Check sheet for the modelled part. Datum: model origin and axes. Units: mm. A direction names the side the tool comes from. Round coordinates to 2 decimals unless told otherwise and drop trailing zeros. Write each loop counter-clockwise with the first axis right and the second up, starting at its lowest first coordinate (ties: lowest second). Pieces come first, ordered by that corner, then holes. Notation, with made-up numbers: (52, 11) -> (82, 11) arc R21 ccw to (82, 44) -> close; hole circle Ø11 at (-37, 85.5). An arc over 180 degrees is marked (long way). Write item = value, one per line.
Autodesk Inventor part; units mm, degrees
ref_plane "YZ Plane" through (0, 0, 0) normal (1, 0, 0) x (0, 1, 0)
ref_plane "XZ Plane" through (0, 0, 0) normal (0, 1, 0) x (-1, 0, 0)
ref_plane "XY Plane" through (0, 0, 0) normal (0, 0, 1) x (1, 0, 0)
sketch "Sketch1" plane through (0, 0, 0) normal (0, 1, 0) x (-1, 0, 0)
  line L0 (-9.45, 13.9) -> (9.45, 13.9)
  line L1 (9.45, 13.9) -> (9.45, 12.4)
  line L2 (9.45, 12.4) -> (-9.45, 12.4)
  line L3 (-9.45, 12.4) -> (-9.45, 13.9)
  line L4 (9.45, 12.4) -> (6.45, 12.4)
  line L5 (6.45, 12.4) -> (6.45, -9)
  line L6 (6.45, -9) -> (9.45, -9)
  line L7 (9.45, -9) -> (9.45, 12.4)
  line L8 (-9.45, 12.4) -> (-7.95, 12.4)
  line L9 (-7.95, 12.4) -> (-7.95, -9)
  line L10 (-7.95, -9) -> (-9.45, -9)
  line L11 (-9.45, -9) -> (-9.45, 12.4)
  line L12 (-7.95, -7.6) -> (-9.45, -7.6)
  line L13 (-9.45, -7.6) -> (-9.45, -10.6)
  line L14 (-9.45, -10.6) -> (-7.95, -10.6)
  line L15 (-7.95, -10.6) -> (-7.95, -7.6)
  line L16 (1.45, -9) -> (9.45, -9)
  line L17 (9.45, -9) -> (9.45, -12)
  line L18 (9.45, -12) -> (1.45, -12)
  line L19 (1.45, -12) -> (1.45, -9)
  line L20 (-9.45, -10.6) -> (-7.95, -10.6)
  line L21 (-7.95, -10.6) -> (-7.95, -27.6)
  line L22 (-7.95, -27.6) -> (-9.45, -27.6)
  line L23 (-9.45, -27.6) -> (-9.45, -10.6)
  line L24 (9.45, -12) -> (6.45, -12)
  line L25 (6.45, -12) -> (6.45, -27.6)
  line L26 (6.45, -27.6) -> (9.45, -27.6)
  line L27 (9.45, -27.6) -> (9.45, -12)
  line L28 (-7.95, -27.6) -> (-19.45, -27.6)
  line L29 (-19.45, -27.6) -> (-19.45, -30.6)
  line L30 (-19.45, -30.6) -> (-7.95, -30.6)
  line L31 (-7.95, -30.6) -> (-7.95, -27.6)
  line L32 (6.45, -27.6) -> (19.45, -27.6)
  line L33 (19.45, -27.6) -> (19.45, -30.6)
  line L34 (19.45, -30.6) -> (6.45, -30.6)
  line L35 (6.45, -30.6) -> (6.45, -27.6)
  line L36 (-14.45, -26) -> (-14.45, -42) construction
  line L37 (14.45, -27) -> (14.45, -42) construction
  point P0 (0, 0)
  point P1 (0, 12.4)
  dimension "d0" = 1.5
  dimension "d1" = 3
  dimension "d2" = 1.5
  dimension "d3" = 3
  dimension "d4" = 3
  dimension "d5" = 0
  dimension "d6" = 5
  dimension "d7" = 14.4
  dimension "d8" = 21.4
  dimension "d9" = 20
  dimension "d12" = 0
  dimension "d13" = 0
  dimension "d20" = 17
  dimension "d21" = 10
  dimension "d22" = 1.5
  dimension "d23" = 3
  dimension "d24" = 10
  dimension "d25" = 3
  dimension "d26" = 3
  dimension "d33" = 5
  dimension "d34" = 5
  dimension "d35" = 28.9
extrude "Extrusion1" add sketch "Sketch1" along normal blind 10
sketch "Sketch6" plane through (19.45, 0, -30.6) normal (0, 0, -1) x (-1, 0, 0)
  line L0 (0, 10) -> (11.5, 10)
  line L1 (0, 0) -> (10, 0)
  line L2 (10, 0) -> (10, 10)
  line L3 (10, 10) -> (0, 10)
  line L4 (0, 10) -> (0, 0)
  circle A0 centre (5, 5) radius 2.25
  point P0 (19.45, 0)
  dimension "d27" = 4.5
sketch "Sketch7" plane through (-6.45, 0, -30.6) normal (0, 0, -1) x (-1, 0, 0)
  line L0 (0, 10) -> (13, 10)
  line L1 (13, 0) -> (3, 0)
  line L2 (3, 0) -> (3, 10)
  line L3 (3, 10) -> (13, 10)
  line L4 (13, 10) -> (13, 0)
  circle A0 centre (8, 5) radius 2.25
  point P0 (-6.45, 0)
  dimension "d28" = 4.5
extrude "Extrusion4" cut sketch "Sketch6" against normal blind 4 contours A0
extrude "Extrusion5" cut sketch "Sketch7" against normal blind 4 contours A0
sketch "Sketch8" plane through (0, 0, 0) normal (0, -1, 0) x (1, 0, 0)
  line L0 (2.9056, 16.2719) -> (14.45, 16.2719)
  line L1 (14.45, 16.2719) -> (14.45, -17.7657)
  line L2 (14.45, -17.7657) -> (2.9056, -17.7657)
  line L3 (2.9056, -17.7657) -> (2.9056, 16.2719)
  point P0 (0, 0)
extrude "Extrusion6" cut sketch "Sketch8" against normal blind 5
equation "\"sp\" = 0.4"
properties part number "MotorMount"
(1) Material ranges on L1, parallel to X at y = 7.75, z = -5.5; L2, parallel to Y at x = -14.45, z = -28.75; L3, parallel to Z at x = -17, y = 1.5, recorded low to high. Write a range as [from, to].
Worked answers:
L1 = [-9.45, -6.45], [7.95, 9.45]
L2 = [0, 2.75], [7.25, 10]
L3 = [-30.6, -27.6]
(2) Sectioned sample at A-A on x = -14.45. Enter the section's corners in (y, z), then the cut area to 3 significant figures.
Worked answers:
outline = (0, -30.6) -> (2.75, -30.6) -> (2.75, -27.6) -> (0, -27.6) -> close; (7.25, -30.6) -> (10, -30.6) -> (10, -27.6) -> (7.25, -27.6) -> close
area = 16.5 mm²
(3) Access from +Z, -Z, +X, -X, +Y, -Y to the whole of each face (thin tool, end or side, straight path). Record for faces 1 (the flat face through (-4, 5, -9)), 2 (the flat face through (-4, 5, -12)), 3 (the flat face through (9, 2, -17.766)), 4 (the flat face through (12, 5, -27.6)).
Worked answers:
face_1 = +Y, -Y
face_2 = -Z, +Y, -Y
face_3 = +Z, +X, -Y
face_4 = +Z, +X, +Y, -Y
(4) Sectioned sample at B-B on z = 0.5. Enter the section's corners in (x, y), then the cut area to 3 significant figures.
Worked answers:
outline = (-9.45, 0) -> (-6.45, 0) -> (-6.45, 10) -> (-9.45, 10) -> close; (7.95, 5) -> (9.45, 5) -> (9.45, 10) -> (7.95, 10) -> close
area = 37.5 mm²
(5) Go/stop test with flat-tipped pins: P1, Ø4, axis at y = 2, z = -1.5, coming from the -X side; P2, Ø4, axis at x = 14.45, y = 5, coming from the -Z side; P3, Ø2.5, axis at x = -4, y = 5.5, coming from the -Z side; P4, Ø3, axis at y = 5.5, z = -12.5, coming from the +X side. Record where each tip stops, or that it passes through.
Worked answers:
P1 = -9.45
P2 = through
P3 = -12
P4 = 9.45
(6) Sectioned sample at C-C on y = 1.5. Enter the section's corners in (x, z).
Worked answers:
outline = (-19.45, -30.6) -> (-6.45, -30.6) -> (-6.45, -12) -> (-1.45, -12) -> (-1.45, -9) -> (-6.45, -9) -> (-6.45, 12.4) -> (2.91, 12.4) -> (2.91, 13.9) -> (-9.45, 13.9) -> (-9.45, -27.6) -> (-19.45, -27.6) -> close; (7.95, -30.6) -> (19.45, -30.6) -> (19.45, -27.6) -> (9.45, -27.6) -> (9.45, -17.77) -> (7.95, -17.77) -> close
(7) Sectioned sample at D-D on y = 5.5. Enter the section's corners in (x, z), then the cut area to 3 significant figures.
Worked answers:
outline = (-19.45, -30.6) -> (-16.64, -30.6) -> (-16.64, -27.6) -> (-19.45, -27.6) -> close; (-12.26, -30.6) -> (-6.45, -30.6) -> (-6.45, -12) -> (-1.45, -12) -> (-1.45, -9) -> (-6.45, -9) -> (-6.45, 12.4) -> (7.95, 12.4) -> (7.95, -30.6) -> (12.26, -30.6) -> (12.26, -27.6) -> (9.45, -27.6) -> (9.45, 13.9) -> (-9.45, 13.9) -> (-9.45, -27.6) -> (-12.26, -27.6) -> close; (16.64, -30.6) -> (19.45, -30.6) -> (19.45, -27.6) -> (16.64, -27.6) -> close
area = 271 mm²
(8) Release check for a two-part mould opening along Y. For faces 5 (the flat face through (-12, 5, -27.6)), 6 (the cylindrical face through (12.304, 5.676, -29.121)), 7 (the flat face through (-8, 0, -10)) record: pulls with the +Y half, pulls with the -Y half, needs draft (parallel to the pull), parting line crosses it, or undercut.
Worked answers:
face_5 = needs draft
face_6 = undercut
face_7 = pulls with the -Y half
